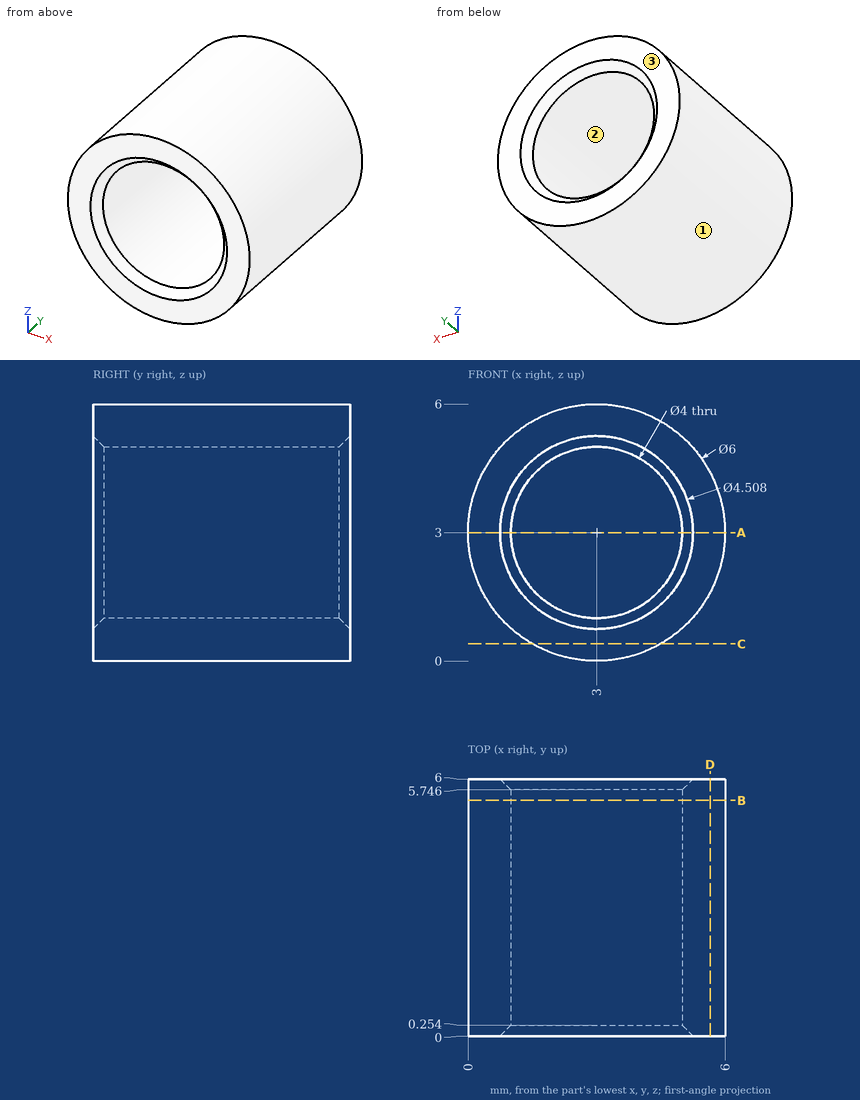
Drawing for the job (mm, zero at the part's lowest x, y, z). Coordinates: 2 decimals unless noted, no trailing zeros. Order: outer loops, then holes, each group sorted by start corner. A loop starts at its lowest first (then second) coordinate and runs counter-clockwise, first axis right, second up. Notation, with made-up numbers: (37, 12) -> (93, 12) arc R20 cw to (93, 19) -> close; hole circle Ø3 at (35, -6.5). An arc over 180 degrees is marked (long way). Return JSON: item names as keys, results as strings.
Item 1: Slice it at C-C (z = 0.4). Write the cut outline in (x, y), then the cut area to 3 significant figures.
Model answer:
{"outline": "(1.5, 0) -> (4.5, 0) -> (4.5, 6) -> (1.5, 6) -> close", "area": "18.0 mm²"}
Item 2: Pin check, flat tip, straight feed: P1, Ø3, axis at x = 2, y = 5, coming from the +Z side. Stop position of the tip, or through.
Model answer:
{"P1": "stops at z = 6"}
Item 3: Slice it at A-A (z = 3). Write the cut outline in (x, y), then the cut area to 3 significant figures.
Model answer:
{"outline": "(0, 0) -> (0.75, 0) -> (1, 0.25) -> (1, 5.75) -> (0.75, 6) -> (0, 6) -> close; (5, 0.25) -> (5.25, 0) -> (6, 0) -> (6, 6) -> (5.25, 6) -> (5, 5.75) -> close", "area": "11.9 mm²"}
Item 4: Slice it at B-B (y = 5.5). Write the cut outline in (x, z), then the cut area to 3 significant figures.
Model answer:
{"outline": "circle Ø6 at (3, 3); hole circle Ø4 at (3, 3)", "area": "15.7 mm²"}
Item 5: Slice it at D-D (x = 5.65). Write the cut outline in (y, z), then the cut area to 3 significant figures.
Model answer:
{"outline": "(0, 1.59) -> (6, 1.59) -> (6, 4.41) -> (0, 4.41) -> close", "area": "16.9 mm²"}
Item 6: Mould opens along Z. For the marked faces 1, 2 and 3 say: pulls with the +Z half, pulls with the -Z half, needs draft (parallel to the pull), parting line crosses it, or undercut.
Model answer:
{"face 1": "parting line crosses it", "face 2": "undercut", "face 3": "needs draft"}
Item 7: Wall check: line 1 along X through (y, z) = (3.8, 3); line 2 along Z through (x, y) = (2.75, 5.05); line 3 along Z through (x, y) = (4.45, 1.7). Give the ranges that are in metal, low to high. Write a range as from..to.
Model answer:
{"line 1": "x = 0..1, 5..6", "line 2": "z = 0.01..1.02, 4.98..5.99", "line 3": "z = 0.37..1.62, 4.38..5.63"}
